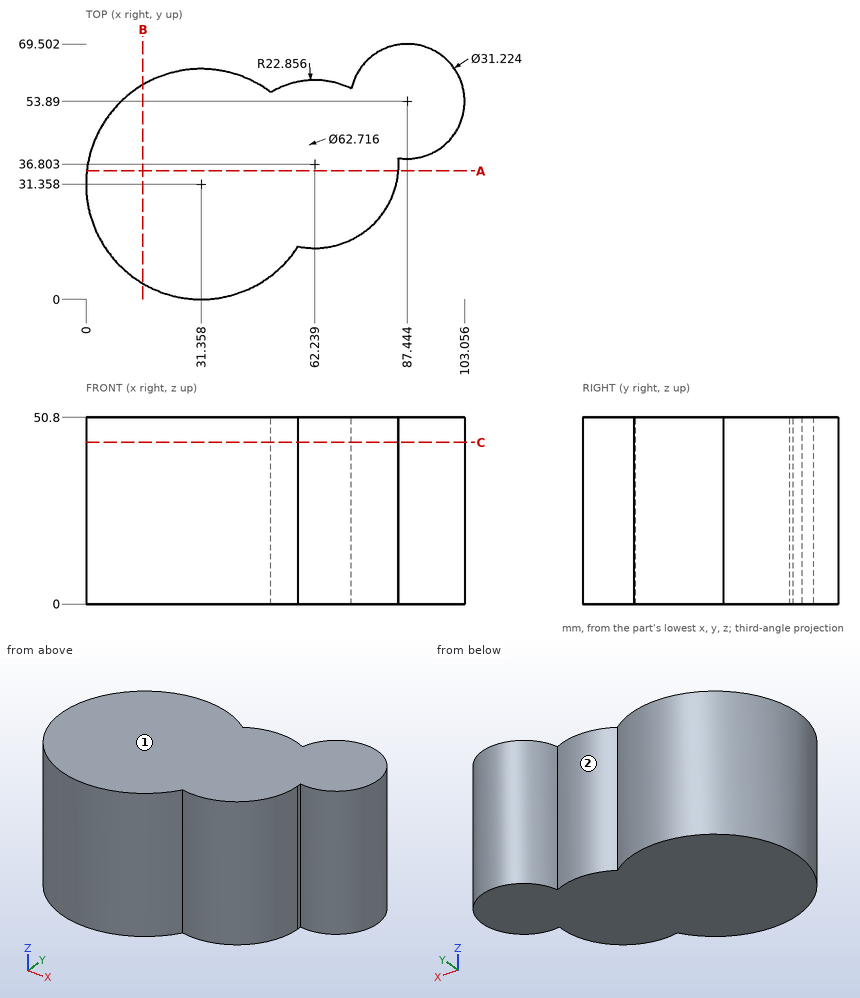
Part print with two shaded views. Sizes in mm from the minimum x, y, z corner. Round coordinates to 2 decimals unless told otherwise and drop trailing zeros. Order: outer loops, then holes, each group sorted by start corner. A loop starts at its lowest first (then second) coordinate and runs counter-clockwise, first axis right, second up. Notation, with made-up numbers: M 32.25,86 L 43.25,86 A16 cw 43.25,113 Z; hole C 50.5,-37.75 d9. An arc over 180 degrees is marked long. Use CSV: the item, a comma, the result in double quotes. Start each with the question number.
(1) Mould opens along X. For the marked faces 1 and 2 say: +X half, -X half, draft (parallel to the pull), parting line (faces both ways), or undercut.
(2) Drill centre lines: probe 1 along Y at (x, z) = (18, 35.5); probe 2 along X at (y, z) = (11, 45) (1 decimal); probe 3 along Y at (x, z) = (92, 39). Where is each one in solid material? Low to high.
(3) Cut at C-C on z = 44. List the corners of the cut face in (x, y) (1 decimal).
(4) Flat gauge pins, fed straight in: P1, Ø1, axis at x = 37, z = 9.5, coming from the +Y side; P2, Ø5, axis at y = 42.5, z = 35.5, coming from the +X side; P3, Ø10, axis at y = 49, z = 33.5, coming from the +X side; P4, Ø4, axis at y = 47.5, z = 30, coming from the -X side. Where does each tip first touch, or does it go through?
(5) Cut at B-B on x = 15.5. List the corners of the cut face in (y, z) (1 decimal).
(6) Cut at A-A on y = 35. List the corners of the cut face in (x, z) (1 decimal).
Findings:
1,face 1,"draft"
1,face 2,"undercut"
2,probe 1,"y = 2.99 to 59.73"
2,probe 2,"x = 7.5 to 55.2"
2,probe 3,"y = 38.96 to 68.82"
3,outline,"M 50.3,56.3 A31.4 ccw long 57.7,14.4 A22.9 ccw 85,38.5 A15.6 ccw long 72.2,57.4 A22.9 ccw Z"
4,P1,"stops at y = 62.29"
4,P2,"stops at x = 100.28"
4,P3,"stops at x = 103.06"
4,P4,"stops at x = 3.37"
5,outline,"M 4.3,0 L 58.4,0 L 58.4,50.8 L 4.3,50.8 Z"
6,outline,"M 0.2,0 L 85,0 L 85,50.8 L 0.2,50.8 Z"
